The listing builds one solid part. Answer for the finished solid, in the listing's coordinates (mm). Coordinates: 2 decimals unless noted, no trailing zeros. Write each loop counter-clockwise with the first axis right and the second up, starting at its lowest first coordinate (ties: lowest second). Pieces come first, ordered by that corner, then holes.
from build123d import *

# Parameters (mm, degrees)
SKETCH1_R            = 10.95
SKETCH1_R_2          = 3.175
BOSS_EXTRUDE1_DEPTH  = 3
M3_CLEARANCE_HOLE1_D = 3.2


with BuildPart() as part:
    # Sketch1 → Boss-Extrude1 (new body)
    with BuildSketch(Plane.XY):
        Circle(SKETCH1_R)
        Circle(SKETCH1_R_2, mode=Mode.SUBTRACT)
    extrude(amount=BOSS_EXTRUDE1_DEPTH)

    # M3 Clearance Hole1 (through all)
    with Locations(Plane.XY.offset(3)):
        with Locations((0, 6.2), (-5.369357503, -3.1), (5.369357503, -3.1)):
            Hole(M3_CLEARANCE_HOLE1_D / 2)


solid = part.part
Q1. The part is cut by section C-C, the plane y = 0. Write down the section's boundary in (x, z) (3 decimals), then the cut area to 4 significant figures.
Answers below:
outline: (-10.95, 0) - (-3.175, 0) - (-3.175, 3) - (-10.95, 3) - close; (3.175, 0) - (10.95, 0) - (10.95, 3) - (3.175, 3) - close
area: 46.65 mm2
Q2. The part is cut by section D-D, the plane x = 6.5. Write down the section's boundary in (y, z).
Answers below:
outline: (-8.81, 0) - (-4.23, 0) - (-4.23, 3) - (-8.81, 3) - close; (-1.97, 0) - (8.81, 0) - (8.81, 3) - (-1.97, 3) - close
Q3. Find the intervals of material crossed by probe 1 along Y at (x, z) = (0, 2) (3 decimals); probe 2 along Y at (x, z) = (-0.5, 2.5); probe 3 along X at (y, z) = (0.5, 0.85), in increasing order.
Answers below:
probe 1: y = -10.95 to -3.175, 3.175 to 4.6, 7.8 to 10.95
probe 2: y = -10.94 to -3.14, 3.14 to 4.68, 7.72 to 10.94
probe 3: x = -10.94 to -3.14, 3.14 to 10.94
Q4. The part is cut by section A-A, the plane x = 0. Write down the section's boundary in (y, z) (3 decimals), then the cut area to 4 significant figures.
Answers below:
outline: (-10.95, 0) - (-3.175, 0) - (-3.175, 3) - (-10.95, 3) - close; (3.175, 0) - (4.6, 0) - (4.6, 3) - (3.175, 3) - close; (7.8, 0) - (10.95, 0) - (10.95, 3) - (7.8, 3) - close
area: 37.05 mm2
Q5. Given pin 1 (5 mm diameter, centred on x = 0, y = 0, fed in from -Z); pin 2 (1 mm diameter, centred on x = 4.5, z = 2.5, fed in from -Y); pin 3 (1 mm diameter, centred on x = -6, z = 0.5, fed in from -Y), each flat-ended and moving along its own axis, determine where each tip first touches the part or whether it passes through.
Answers below:
pin 1: passes through
pin 2: stops at y = -10.19
pin 3: stops at y = -9.47
Q6. The part is cut by section B-B, the plane z = 1.3. Write down the section's boundary in (x, y) (3 decimals).
Answers below:
outline: circle Ø21.9 at (0, 0); hole circle Ø3.2 at (-5.369, -3.1); hole circle Ø6.35 at (0, 0); hole circle Ø3.2 at (0, 6.2); hole circle Ø3.2 at (5.369, -3.1)
Q7. Determine the mould class of faces 1 (the face through (-0.69, -3.1, 1.48)), 2 (the face through (-3, -2, 3)), 3 (the face through (-8.69, -6.66, 1.48)) for opening direction Y: released by +Y, released by -Y, zero draft, split by the parting line, or undercut.
Answers below:
face 1: undercut
face 2: zero draft
face 3: split by the parting line
